from build123d import *

# Parameters (mm, degrees)
F1_DEPTH = 76.2
F3_D     = 38.1


with BuildPart() as f1:
    # F0 (on Front) → F1 (new body)
    with BuildSketch(Plane.XZ):
        Polygon((-47.625, 52.3875), (-47.625, -52.3875), (47.625, -52.3875), (47.625, 52.3875), (28.575, 52.3875), (28.575, -30.1625), (-28.575, -30.1625), (-28.575, 52.3875), align=None)
    extrude(amount=F1_DEPTH)

    # F3 (through all)
    with Locations(Plane(origin=(-47.625, 0, 0), x_dir=(0, -1, 0), z_dir=(-1, 0, 0))):
        with Locations((38.1, 20.6375)):
            Hole(F3_D / 2)


solid = f1.part
CAD build for the part. Positions are in the model's coordinates, mm. A direction names the side the tool comes from. Give positions to 0.01 mm unless a question says otherwise; leave off trailing zeros. Loops run counter-clockwise (first coordinate to the right, second up) from the corner with the lowest first, then second, coordinate; pieces in that order, holes last. Notation, with made-up numbers: M -3.75,1.5 L 29.25,1.5 A15 cw 29.25,17.5 Z; hole C 13.25,63.5 d11. An arc over 180 degrees is marked long. Answer in a Markdown table with one row per item. Add a question column.
Item 1: Band-saw the part on C-C on z = 30. Give the cut face in (x, y) (3 decimals), then the cut area to 3 significant figures.
Item 2: Band-saw the part on A-A on z = 45. Give the cut face in (x, y) (3 decimals), then the cut area to 3 significant figures.
Item 3: Probe probe 1 along X at (y, z) = (-18, 34) (3 decimals); probe 2 along Z at (x, y) = (-36, -38.1); probe 3 along Z at (x, y) = (-21.5, -27). List the from-to ranges inside material, lowest first.
Item 4: Band-saw the part on D-D on y = -4.5. Give the cut face in (x, z) (1 decimal), then the cut area to 3 significant figures.
Item 5: Mould opens along X. For faces 3 (the face through (-38, -38, 52.388)), 4 (the face through (-28.575, -38, 1)), 5 (the face through (-47.625, -38, 1)) say: +X half, -X half, draft (parallel to the pull), parting line (faces both ways), or undercut.
Item 6: Band-saw the part on B-B on y = -38.1. Give the cut face in (x, z) (1 decimal), then the cut area to 3 significant figures.
Item 7: Drop a flat-ended pin along its axis: P1, Ø3, axis at x = 8, y = -15, coming from the +Z side. Give the stop position or say it passes through.
Item 8: Tool access for faces 1 (the face through (-37.97, -42.23, 2.04)), 2 (the face through (28.575, -29, 3)): list every direction of +Z, -Z, +X, -X, +Y, -Y with a clear straight run to the whole face (end or side of a thin tool).
Reply:
| question | item | result |
|---|---|---|
| 1 | outline | M -47.625,-76.2 L -28.575,-76.2 L -28.575,-54.691 L -47.625,-54.691 Z; M -47.625,-21.509 L -28.575,-21.509 L -28.575,0 L -47.625,0 Z; M 28.575,-76.2 L 47.625,-76.2 L 47.625,-54.691 L 28.575,-54.691 Z; M 28.575,-21.509 L 47.625,-21.509 L 47.625,0 L 28.575,0 Z |
| 1 | area | 1,640 mm^2 |
| 2 | outline | M -47.625,-76.2 L -28.575,-76.2 L -28.575,0 L -47.625,0 Z; M 28.575,-76.2 L 47.625,-76.2 L 47.625,0 L 28.575,0 Z |
| 2 | area | 2,900 mm^2 |
| 3 | probe 1 | x = -47.625 to -28.575, 28.575 to 47.625 |
| 3 | probe 2 | z = -52.39 to 1.59, 39.69 to 52.39 |
| 3 | probe 3 | z = -52.39 to -30.16 |
| 4 | outline | M -47.6,-52.4 L 47.6,-52.4 L 47.6,52.4 L 28.6,52.4 L 28.6,-30.2 L -28.6,-30.2 L -28.6,52.4 L -47.6,52.4 Z |
| 4 | area | 5,260 mm^2 |
| 5 | face 3 | draft |
| 5 | face 4 | undercut |
| 5 | face 5 | -X half |
| 6 | outline | M -47.6,-52.4 L 47.6,-52.4 L 47.6,1.6 L 28.6,1.6 L 28.6,-30.2 L -28.6,-30.2 L -28.6,1.6 L -47.6,1.6 Z; M -47.6,39.7 L -28.6,39.7 L -28.6,52.4 L -47.6,52.4 Z; M 28.6,39.7 L 47.6,39.7 L 47.6,52.4 L 28.6,52.4 Z |
| 6 | area | 3,810 mm^2 |
| 7 | P1 | stops at z = -30.16 |
| 8 | face 1 | +X, -X |
| 8 | face 2 | +Z, +Y, -Y |
